```python
from build123d import *

# Parameters (mm, degrees)
F0_W        = 18
F0_H        = 9.2
F0_W_2      = 15.6
F0_H_2      = 3.2
F1_DEPTH    = 0.9
F2_T1_DEPTH = 23.6577025735
F2_T3_DEPTH = 14.8577025735
F3_R        = 1


# Not quite as in the source:
# - a fillet or chamfer that OpenCascade refuses, or shapes differently, is made with other operations: its cross-section is extruded or revolved along the edge and cut away or added


with BuildPart() as f1:
    # F0 (on Top) → F1 (new body)
    with BuildSketch(Plane.XY):
        Rectangle(F0_W, F0_H)
        with Locations((0, -1.8)):
            Rectangle(F0_W_2, F0_H_2, mode=Mode.SUBTRACT)
        with Locations((0, 1.8)):
            Rectangle(F0_W_2, F0_H_2, mode=Mode.SUBTRACT)
    extrude(amount=F1_DEPTH)

    # F2: chamfer of 1.1 on 4 edges, made by hand

    # F2_s2 → F2_t1 (cut)
    with BuildSketch(Plane.YZ.offset(-11.8288512868)):
        Polygon((-4.6, -0.2), (-3.5, 0.9), (-4.6, 0.9), align=None)
        Polygon((4.6, -0.2), (3.5, 0.9), (4.6, 0.9), align=None)
    extrude(amount=F2_T1_DEPTH, mode=Mode.SUBTRACT)

    # F2_s4 → F2_t3 (cut)
    with BuildSketch(Plane.XZ.offset(-7.4288512868)):
        Polygon((-9, -0.2), (-7.9, 0.9), (-9, 0.9), align=None)
        Polygon((9, -0.2), (7.9, 0.9), (9, 0.9), align=None)
    extrude(amount=F2_T3_DEPTH, mode=Mode.SUBTRACT)

    # F3
    f3_edges = [f1.edges().sort_by_distance(p)[0] for p in [
        (-7.8, 3.4, 0.45),
        (-7.8, -0.2, 0.45),
        (7.8, 0.2, 0.45),
        (7.8, -3.4, 0.45),
        (7.8, 3.4, 0.45),
        (7.8, -0.2, 0.45),
        (-7.8, 0.2, 0.45),
        (-7.8, -3.4, 0.45),
        (-8.35, -3.95, 0.45),
        (8.35, -3.95, 0.45),
        (8.35, 3.95, 0.45),
        (-8.35, 3.95, 0.45),
    ]]
    fillet(f3_edges, radius=F3_R)


solid = f1.part
```
Here's how the part is built. I have some questions about the finished solid (model axes, mm). A direction names the side the tool comes from. Coordinates: 2 decimals unless noted, no trailing zeros. Write each loop counter-clockwise with the first axis right and the second up, starting at its lowest first coordinate (ties: lowest second). Pieces come first, ordered by that corner, then holes. Notation, with made-up numbers: (-10.5, 40.5) -> (32.5, 40.5) arc R14 cw to (32.5, 50.5) -> close; hole circle Ø8 at (-18, 37). An arc over 180 degrees is marked (long way). Use a Markdown table: item, result. Add a question column.
(1) If we section it at B-B, the plane y = 2: Write out the boundary of the cut face in (x, z), and give its area (3 significant figures).
(2) If we section it at D-D, the plane z = 0.7: State how many separate pieces and enclosed holes the cut face has, and give its area (3 significant figures).
(3) We'd pull the mould along X, two halves only. Please class faces 3 (the cylindrical face through (-8.138, -3.728, 0.477)), 4 (the flat face through (-0.1, 0.2, 0.4)), 5 (the flat face through (7.8, 1.8, 0.4)), 6 (the cylindrical face through (8.138, -3.728, 0.477)): +X half, -X half, draft (parallel to the pull), parting line (faces both ways), or undercut.
(4) If we section it at A-A, the plane x = 3.25: Write out the boundary of the cut face in (y, z).
(5) Please list where these lines run through material, in increasing order: line 1 (Y direction, x = -6.25, z = 0.4); line 2 (Y direction, x = 6, z = 0.45); line 3 (X direction, y = 2, z = 0.75).
(6) For faces 1 (the flat face through (-8.4, 0.1, 0.4)), 2 (the cylindrical face through (7.499, -3.115, 0.456)), which set-ups out of +Z, -Z, +X, -X, +Y, -Y let a thin tool reach every point of the face, with its end or its side?
(7) If we section it at C-C, the plane y = 1: Write out the boundary of the cut face in (x, z).
Outcome:
| question | item | result |
|---|---|---|
| 1 | outline | (-8.8, 0) -> (-7.8, 0) -> (-7.8, 0.9) -> (-7.9, 0.9) -> close; (7.8, 0) -> (8.8, 0) -> (7.9, 0.9) -> (7.8, 0.9) -> close |
| 1 | area | 0.990 mm^2 |
| 2 | separate pieces | 1 |
| 2 | enclosed holes | 2 |
| 2 | area | 21.4 mm^2 |
| 3 | face 3 | -X half |
| 3 | face 4 | undercut |
| 3 | face 5 | undercut |
| 3 | face 6 | +X half |
| 4 | outline | (-4.4, 0) -> (-3.4, 0) -> (-3.4, 0.9) -> (-3.5, 0.9) -> close; (-0.2, 0) -> (0.2, 0) -> (0.2, 0.9) -> (-0.2, 0.9) -> close; (3.4, 0) -> (4.4, 0) -> (3.5, 0.9) -> (3.4, 0.9) -> close |
| 5 | line 1 | y = -4 to -3.4, -0.2 to 0.2, 3.4 to 4 |
| 5 | line 2 | y = -3.95 to -3.4, -0.2 to 0.2, 3.4 to 3.95 |
| 5 | line 3 | x = -8.05 to -7.8, 7.8 to 8.05 |
| 6 | face 1 | +Z, -X, +Y, -Y |
| 6 | face 2 | +Z, -Z |
| 7 | outline | (-8.8, 0) -> (-7.78, 0) -> (-7.78, 0.9) -> (-7.9, 0.9) -> close; (7.78, 0) -> (8.8, 0) -> (7.9, 0.9) -> (7.78, 0.9) -> close |
